For this review, use the dimensioned drawing (mm, ordinates from the lowest corner) and the shaded views. A direction names the side the tool comes from. Coordinates: 2 decimals unless noted, no trailing zeros. Loops run counter-clockwise (first coordinate to the right, second up) from the corner with the lowest first, then second, coordinate; pieces in that order, holes last. Notation, with made-up numbers: M 54,0.25 L 84,0.25 A37 cw 84,36.25 Z; hole C 17.25,-30.75 d11. An arc over 180 degrees is marked long. Use CSV: the item, a comma, the result in double quotes. Start each with the question number.
1. Add section D-D, the plane z = 10.25. Write out the cut boundary in (x, y).
2. Add section A-A, the plane y = 3.1. Write out the cut boundary in (x, z).
3. Draft analysis for pull direction Z (two halves, no side actions). For the marked faces 1, 2 and 3, state which applies: +Z half, -Z half, draft (parallel to the pull), parting line (faces both ways), or undercut.
4. Clearance check with flat-ended pins moving along their axes: P1, Ø2, axis at x = 10.95, z = 19.15, coming from the +Y side; P2, Ø1, axis at y = 2.5, z = 14, coming from the -X side; P3, Ø3, axis at x = 10.95, z = 2.75, coming from the -Y side. State where each tip first meets the part, or that it passes through.
5. Tool access review of the marked faces 4 and 5: name each direction out of +Z, -Z, +X, -X, +Y, -Y from which nothing blocks a thin tool from reaching the whole face with its end or side.
6. Add section C-C, the plane x = 2.75. Write out the cut boundary in (y, z), then the cut area to 3 significant figures.
7. For L1, parallel to Z at x = 10.95, y = 4.4; L2, parallel to X at y = 4.5, z = 10.5; L3, parallel to Y at x = 12.75, z = 18.25, list the stretches that pass through material, from the lowest coordinate up.
8. Add section B-B, the plane z = 19.15. Write out the cut boundary in (x, y), then the cut area to 3 significant figures.
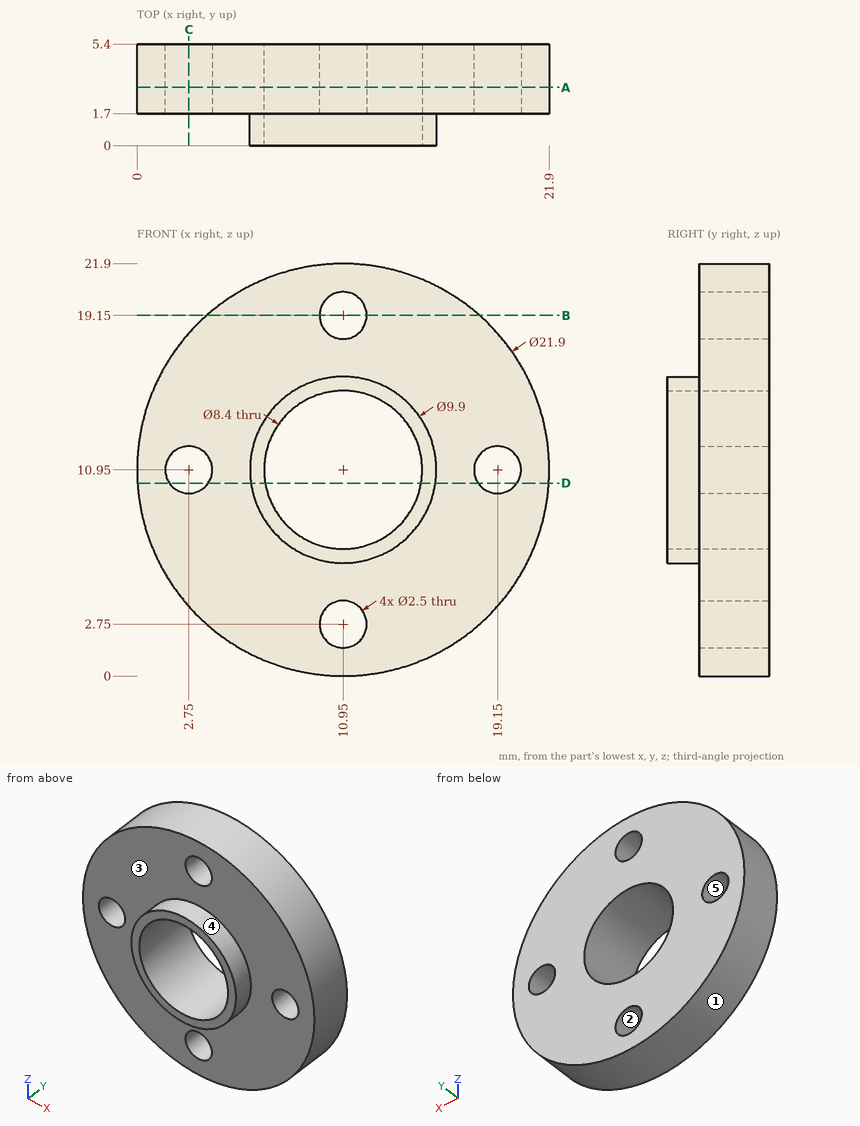
Computed:
1,outline,"M 0.02,1.7 L 1.71,1.7 L 1.71,5.4 L 0.02,5.4 Z; M 3.79,1.7 L 6.05,1.7 L 6.05,0 L 6.81,0 L 6.81,5.4 L 3.79,5.4 Z; M 15.09,0 L 15.85,0 L 15.85,1.7 L 18.11,1.7 L 18.11,5.4 L 15.09,5.4 Z; M 20.19,1.7 L 21.88,1.7 L 21.88,5.4 L 20.19,5.4 Z"
2,outline,"C 10.95,10.95 d21.9; hole C 2.75,10.95 d2.5; hole C 10.95,10.95 d8.4; hole C 10.95,2.75 d2.5; hole C 10.95,19.15 d2.5; hole C 19.15,10.95 d2.5"
3,face 1,"parting line"
3,face 2,"undercut"
3,face 3,"draft"
4,P1,"passes through"
4,P2,"stops at x = 0.3"
4,P3,"stops at y = 1.7"
5,face 4,"-Y"
5,face 5,"+Y, -Y"
6,outline,"M 1.7,3.69 L 5.4,3.69 L 5.4,9.7 L 1.7,9.7 Z; M 1.7,12.2 L 5.4,12.2 L 5.4,18.21 L 1.7,18.21 Z"
6,area,"44.5 mm^2"
7,L1,"z = 0 to 1.5, 4 to 6.75, 15.15 to 17.9, 20.4 to 21.9"
7,L2,"x = 0.01 to 1.58, 3.92 to 6.77, 15.13 to 17.98, 20.32 to 21.89"
7,L3,"y = 1.7 to 5.4"
8,outline,"M 3.69,1.7 L 9.7,1.7 L 9.7,5.4 L 3.69,5.4 Z; M 12.2,1.7 L 18.21,1.7 L 18.21,5.4 L 12.2,5.4 Z"
8,area,"44.5 mm^2"
